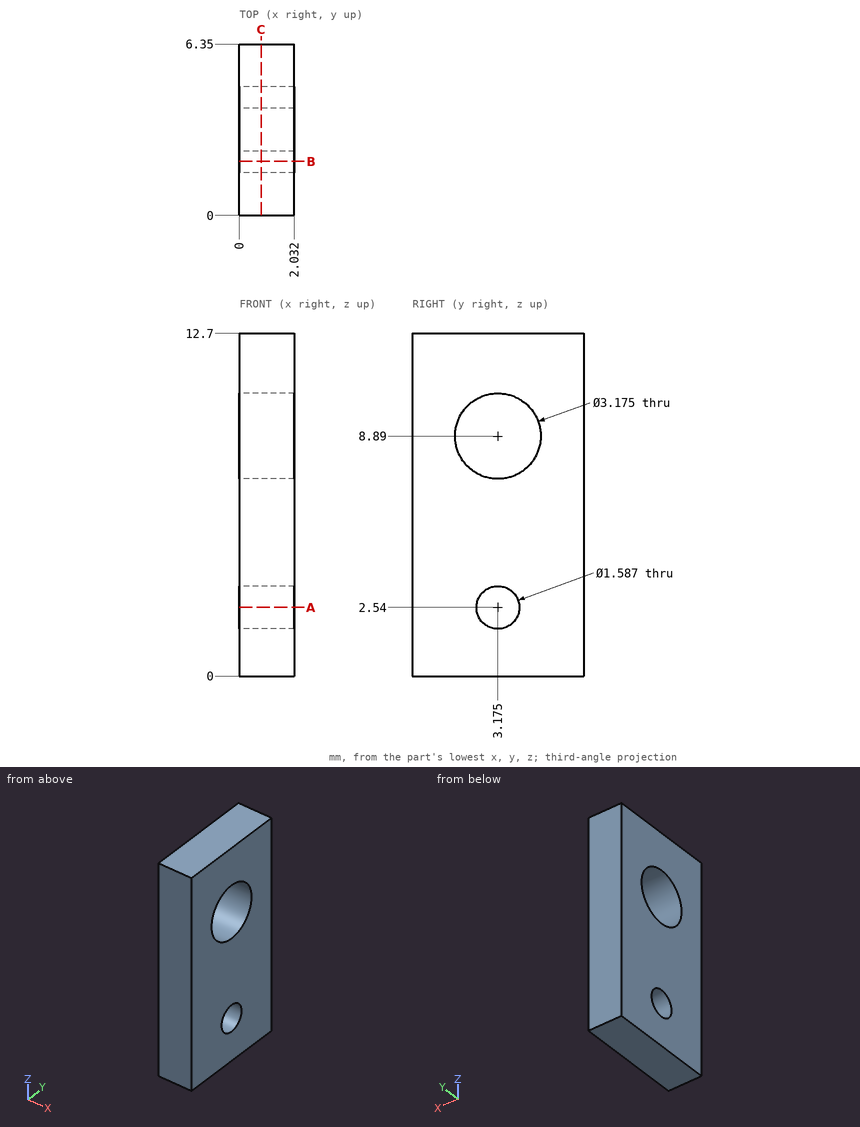
Part print with two shaded views. Sizes in mm from the minimum x, y, z corner. Round coordinates to 2 decimals unless told otherwise and drop trailing zeros. Loops run counter-clockwise (first coordinate to the right, second up) from the corner with the lowest first, then second, coordinate; pieces in that order, holes last. Notation, with made-up numbers: (79, 75.25) - (95, 75.25) arc R34 cw to (95, 109.25) - close; hole circle Ø2 at (47, 29). An arc over 180 degrees is marked (long way). Answer as a JSON object with one key per item and string values.
Item 1: Wall check: L1, parallel to Y at x = 0.6, z = 2.54; L2, parallel to Y at x = 0.6, z = 8.89; L3, parallel to Z at x = 0.4, y = 3 (1 decimal). Give the ranges that are in metal, low to high.
Output:
{"L1": "0 to 2.38, 3.97 to 6.35", "L2": "0 to 1.59, 4.76 to 6.35", "L3": "0 to 1.8, 3.3 to 7.3, 10.5 to 12.7"}
Item 2: Band-saw the part on B-B on y = 2. List the corners of the cut face in (x, z).
Output:
{"outline": "(0, 0) - (2.03, 0) - (2.03, 7.82) - (0, 7.82) - close; (0, 9.96) - (2.03, 9.96) - (2.03, 12.7) - (0, 12.7) - close"}
Item 3: Band-saw the part on A-A on z = 2.54. List the corners of the cut face in (x, y).
Output:
{"outline": "(0, 0) - (2.03, 0) - (2.03, 2.38) - (0, 2.38) - close; (0, 3.97) - (2.03, 3.97) - (2.03, 6.35) - (0, 6.35) - close"}
Item 4: Band-saw the part on C-C on x = 0.8. State how many separate pieces and enclosed holes the cut face has.
Output:
{"separate pieces": "1", "enclosed holes": "2"}
